For this review, take the finished solid that the model builds, in its own axes (mm). A direction names the side the tool comes from. Round coordinates to 2 decimals unless told otherwise and drop trailing zeros. Write each loop counter-clockwise with the first axis right and the second up, starting at its lowest first coordinate (ties: lowest second). Pieces come first, ordered by that corner, then holes. Notation, with made-up numbers: (78.25, 14.5) -> (117.25, 14.5) arc R14 cw to (117.25, 37.5) -> close; hole circle Ø8 at (-24, 46.25). An arc over 180 degrees is marked (long way). Answer in a Markdown table with one row per item. Add a question column.
```python
from build123d import *

# Parameters (mm, degrees)
BOSS_EXTRUDE1_DEPTH     = 15
SKETCH2_R               = 11.1
CUT_EXTRUDE1_DEPTH      = 10
SKETCH3_R               = 5
CUT_EXTRUDE2_DEPTH      = 10
CUT_EXTRUDE_THIN7_DEPTH = 62


with BuildPart() as part:
    # Sketch1 → Boss-Extrude1 (new body)
    with BuildSketch(Plane.XY):
        with BuildLine():
            Line((5.505816945, 85.326012217), (5.307768654, 85.393580353))
            ThreePointArc((5.307768654, 85.393580353), (-2.005055015, 101.475976607), (13.940536847, 109.082484312))
            Line((13.940536847, 109.082484312), (40.538740524, 99.7887516))
            Line((40.538740524, 99.7887516), (48.129208704, 80.495248668))
            Line((48.129208704, 80.495248668), (17.636215156, 25.115965593))
            ThreePointArc((17.636215156, 25.115965593), (18.579608232, 12.6739017), (11.964278199, 2.09409296))
            Line((11.964278199, 2.09409296), (12.243619866, -31.678974911))
            ThreePointArc((12.243619866, -31.678974911), (0.468324559, -67.537617109), (-12.751239862, -32.185913949))
            Line((-12.751239862, -32.185913949), (-13.03091257, 1.603476045))
            ThreePointArc((-13.03091257, 1.603476045), (-20.259022529, 22.242640416), (-4.270337109, 37.161843413))
            Line((-4.270337109, 37.161843413), (-0.71558036, 43.617748767))
            Line((-0.71558036, 43.617748767), (5.505816945, 85.326012217))
        make_face()
    extrude(amount=BOSS_EXTRUDE1_DEPTH)

    # Sketch2 → Cut-Extrude1 (cut)
    with BuildSketch(Plane(origin=(0, 0, 0), x_dir=(-1, 0, 0), z_dir=(0, 0, -1))):
        with Locations((0.839707244, 17.458270673)):
            Circle(SKETCH2_R)
        with Locations((-0.062773329, -47.541729327)):
            Circle(SKETCH2_R)
    extrude(amount=-CUT_EXTRUDE1_DEPTH, mode=Mode.SUBTRACT)

    # Sketch3 → Cut-Extrude2 (cut)
    with BuildSketch(Plane(origin=(0, 0, 10), x_dir=(-1, 0, 0), z_dir=(0, 0, -1))):
        with Locations((0.839707244, 17.458270673)):
            Circle(SKETCH3_R)
        with Locations((-0.062773329, -47.541729327)):
            Circle(SKETCH3_R)
    extrude(amount=-CUT_EXTRUDE2_DEPTH, mode=Mode.SUBTRACT)

    # Sketch4 → Cut-Extrude-Thin7 (cut)
    with BuildSketch(Plane(origin=(35.484462303, 101.554777284, 0), x_dir=(0.944031293, -0.329855904, 0), z_dir=(0.329855904, 0.944031293, 0))):
        Polygon((-17.177390776, -0.155952815), (-35.822204189, -5.255346546), (-38.460333018, 4.390392216), (-19.815519606, 9.489785947), align=None)
        Polygon((-36.000883233, -9.902707664), (-17.695137785, -14.971739454), (-20.363805607, -24.609073736), (-38.669551056, -19.540041946), align=None)
    extrude(amount=-CUT_EXTRUDE_THIN7_DEPTH, mode=Mode.SUBTRACT)


solid = part.part
```
1. For L1, parallel to Y at x = 8.5, z = 3.5; L2, parallel to X at y = -2, z = 1; L3, parallel to Y at x = 13, z = 7.5, list the stretches that pass through material, from the lowest coordinate up. Write a range as [from, to].
2. We need section C-C (y = 14.5). Write out the cut boundary in (x, z).
3. The part is to be moulded in two halves that separate along Y. For faces 1 (the flat face through (6, 21, 15)), 2 (the cylindrical face through (0.244, 12.577, 12.465)), 3 (the flat face through (44.28, 90.28, 7.4)), 4 (the flat face through (-3.2, 12.7, 10)), say which applies: pulls with the +Y half, pulls with the -Y half, needs draft (parallel to the pull), parting line crosses it, or undercut.
4. We need section B-B (z = 3.5). Write out the cut boundary in (x, y).
5. Tool access review of faces 5 (the cylindrical face through (1.508, -36.536, 4.93)), 6 (the cylindrical face through (1.16, -67.51, 7.4)), 7 (the flat face through (-2.52, 40.34, 7.4)): name each direction out of +Z, -Z, +X, -X, +Y, -Y from which nothing blocks a thin tool from reaching the whole face with its end or side.
6. Clearance check with flat-ended pins moving along their axes: pin 1 Ø3 at (y, z) = (5, 11) entering from +X; pin 2 Ø18 at (x, y) = (-0.84, 17.46) entering from -Z; pin 3 Ø8 at (y, z) = (46, 8.5) entering from +X. State where each tip first meets the part, or that it passes through.
Response:
| question | item | result |
|---|---|---|
| 1 | L1 | [-65.67, -54.75], [-40.33, 11.46], [23.46, 109.7] |
| 1 | L2 | [-13, 12] |
| 1 | L3 | [-62.79, -32.29], [3.02, 109.37] |
| 2 | outline | (-20.62, 0) -> (-11.54, 0) -> (-11.54, 10) -> (-4.87, 10) -> (-4.87, 15) -> (-20.62, 15) -> close; (3.19, 10) -> (9.86, 10) -> (9.86, 0) -> (18.94, 0) -> (18.94, 15) -> (3.19, 15) -> close |
| 3 | face 1 | needs draft |
| 3 | face 2 | undercut |
| 3 | face 3 | pulls with the +Y half |
| 3 | face 4 | undercut |
| 4 | outline | (-13.03, 1.6) -> (-12.75, -32.19) arc R20 ccw (long way) to (12.24, -31.68) -> (11.96, 2.09) arc R20 ccw to (17.64, 25.12) -> (48.13, 80.5) -> (40.54, 99.79) -> (13.94, 109.08) arc R12.61 ccw to (7.1, 109.47) -> (0.03, 89.24) arc R12.61 ccw to (5.31, 85.39) -> (5.51, 85.33) -> (-0.72, 43.62) -> (-4.27, 37.16) arc R20 ccw to start; hole circle Ø22.2 at (-0.84, 17.46); hole circle Ø22.2 at (0.06, -47.54) |
| 5 | face 5 | -Z |
| 5 | face 6 | +Z, -Z |
| 5 | face 7 | +Z, -Z, -X |
| 6 | pin 1 | x = 15.89 |
| 6 | pin 2 | z = 10 |
| 6 | pin 3 | x = 31.34 |
